The listing builds one solid part. Answer for the finished solid, in the listing's coordinates (mm). A direction names the side the tool comes from. Give positions to 0.01 mm unless a question says otherwise; leave off trailing zeros. Loops run counter-clockwise (first coordinate to the right, second up) from the corner with the lowest first, then second, coordinate; pieces in that order, holes last. Notation, with made-up numbers: M 13,61.25 L 60,61.25 A8 ccw 60,73.25 Z; hole C -0.75,-24 d1. An arc over 180 degrees is marked long. One line per item, written item: value. Start each with the question number.
Q1. Consider L1, parallel to X at y = 1.6, z = -3.75; L2, parallel to Y at x = 3, z = 7.5; L3, parallel to Y at x = -5.75, z = -0.25. Determine where each line is inside the solid, lowest interval first.
Q2. The mould has two halves that part along X. Classify faces 1 (the flat face through (8, 3, -3)), 2 (the cylindrical face through (4.579, 0.641, -5.356)), 3 (the flat face through (8.5, 2, -1)), 4 (the cylindrical face through (0, 1.8, 3.4)): +X half, -X half, draft (parallel to the pull), parting line (faces both ways), or undercut.
Q3. A cutting plane is placed at A-A, the plane y = 2.1. Determine the outline of the cut face in (x, z), and give its area (3 significant figures).
Q4. A cutting plane is placed at D-D, the plane x = -3. Determine the outline of the cut face in (y, z), and give its area (3 significant figures).
Q5. For faces 5 (the flat face through (0, 2, -8.5)), 6 (the flat face through (-8, 3, -3)), 7 (the flat face through (5, 0, -6)), 8 (the cylindrical face through (-6.421, 0.641, 6.144)), 9 (the cylindrical face through (0, 3, -8)), determine the directions among +Z, -Z, +X, -X, +Y, -Y from which every point of the face is accessible in a straight line to the end or side of a thin tool.
Q6. A cutting plane is placed at B-B, the plane x = 0. Determine the outline of the cut face in (y, z).
Q7. A cutting plane is placed at C-C, the plane z = 5.5. Determine the outline of the cut face in (x, y), and give its area (3 significant figures).
Q8. Flat-ended cylindrical pins translate along their axes: pin 1 (1 mm diameter, centred on x = -2.5, z = -6.5, fed in from -Y); pin 2 (4.5 mm diameter, centred on x = -3.5, z = 4.5, fed in from +Y); pin 3 (1.2 mm diameter, centred on x = -8, y = 3, fed in from +Z). Find the tip coordinate at first contact, or state that the pin passes through.
from build123d import *

# Parameters (mm, degrees)
SKETCH1_W           = 17
SKETCH1_H           = 17
BOSS_EXTRUDE1_DEPTH = 3.5
CUT_EXTRUDE1_DEPTH  = 4.5
CUT_EXTRUDE2_DEPTH  = 0.6
SKETCH5_W           = 17
SKETCH5_H           = 6
CUT_EXTRUDE3_DEPTH  = 0.6
SKETCH6_R           = 8
CUT_EXTRUDE4_DEPTH  = 1.2
SKETCH7_OUTSIDE_W   = 23.86
SKETCH7_OUTSIDE_H   = 23.86
SKETCH7_OUTSIDE_R   = 1.25
CUT_EXTRUDE5_DEPTH  = 1.3
CUT_EXTRUDE6_DEPTH  = 1
BOSS_EXTRUDE4_DEPTH = 1


with BuildPart() as part:
    # Sketch1 → Boss-Extrude1 (new body)
    with BuildSketch(Plane(origin=(0, 0, 0), x_dir=(1, 0, 0), z_dir=(0, 1, 0))):
        Rectangle(SKETCH1_W, SKETCH1_H)
    extrude(amount=BOSS_EXTRUDE1_DEPTH)

    # Sketch2 → Cut-Extrude1 (cut, through all)
    with BuildSketch(Plane(origin=(0, 3.5, 0), x_dir=(1, 0, 0), z_dir=(0, 1, 0))):
        Polygon((-8.5, -5.812994231), (-5.812994231, -8.5), (-8.5, -8.5), align=None)
    cut_extrude1 = extrude(amount=-CUT_EXTRUDE1_DEPTH, mode=Mode.SUBTRACT)

    # Mirror1: Cut-Extrude1 across plane
    add(cut_extrude1.mirror(Plane(origin=(0, 0, 0), x_dir=(0, 0, 1), z_dir=(1, 0, 0))), mode=Mode.SUBTRACT)

    # Sketch3 → Cut-Extrude2 (cut)
    with BuildSketch(Plane(origin=(0, 3.5, 0), x_dir=(1, 0, 0), z_dir=(0, 1, 0))):
        Polygon((-8.5, 3), (8.5, 3), (8.5, -5.812994231), (5.812994231, -8.5), (-5.812994231, -8.5), (-8.5, -5.812994231), align=None)
    extrude(amount=-CUT_EXTRUDE2_DEPTH, mode=Mode.SUBTRACT)

    # Sketch5 → Cut-Extrude3 (cut)
    with BuildSketch(Plane(origin=(0, 2.9, 0), x_dir=(1, 0, 0), z_dir=(0, 1, 0))):
        Rectangle(SKETCH5_W, SKETCH5_H)
    extrude(amount=-CUT_EXTRUDE3_DEPTH, mode=Mode.SUBTRACT)

    # Sketch6 → Cut-Extrude4 (cut)
    with BuildSketch(Plane(origin=(0, 3.5, 0), x_dir=(1, 0, 0), z_dir=(0, 1, 0))):
        Circle(SKETCH6_R)
    extrude(amount=-CUT_EXTRUDE4_DEPTH, mode=Mode.SUBTRACT)

    # Sketch7 outside → Cut-Extrude5 (cut)
    with BuildSketch(Plane.XZ):
        Rectangle(SKETCH7_OUTSIDE_W, SKETCH7_OUTSIDE_H)
        with Locations((-5.5, -6.20094747)):
            Circle(SKETCH7_OUTSIDE_R, mode=Mode.SUBTRACT)
        with Locations((-5.5, 5.29905253)):
            Circle(SKETCH7_OUTSIDE_R, mode=Mode.SUBTRACT)
        with Locations((5.5, 5.29905253)):
            Circle(SKETCH7_OUTSIDE_R, mode=Mode.SUBTRACT)
        with Locations((5.5, -6.20094747)):
            Circle(SKETCH7_OUTSIDE_R, mode=Mode.SUBTRACT)
    extrude(amount=-CUT_EXTRUDE5_DEPTH, mode=Mode.SUBTRACT)

    # Sketch8 → Cut-Extrude6 (cut)
    with BuildSketch(Plane.XZ.offset(-1.3)):
        with BuildLine():
            Line((-0.6, -8.5), (0.6, -8.5))
            Line((0.6, -8.5), (0.749551834, -4.175923885))
            ThreePointArc((0.749551834, -4.175923885), (0, -3.4), (-0.749551834, -4.175923885))
            Line((-0.749551834, -4.175923885), (-0.6, -8.5))
        make_face()
    cut_extrude6 = extrude(amount=-CUT_EXTRUDE6_DEPTH, mode=Mode.SUBTRACT)

    # Mirror2: Cut-Extrude6 across plane
    add(cut_extrude6.mirror(Plane.XY), mode=Mode.SUBTRACT)

    # Sketch11 → Boss-Extrude4 (add)
    with BuildSketch(Plane.XZ.offset(-1.3)):
        Polygon((-0.6, -8.5), (0.6, -8.5), (0.634585847, -7.5), (-0.634585847, -7.5), align=None)
    boss_extrude4 = extrude(amount=-BOSS_EXTRUDE4_DEPTH)

    # Mirror3: Boss-Extrude4 across plane
    add(boss_extrude4.mirror(Plane.XY))


solid = part.part
Answer block:
1. L1: -8.5 to -0.63, 0.63 to 8.5
1. L2: 1.3 to 2.9
1. L3: 1.3 to 2.3
2. face 1: draft
2. face 2: undercut
2. face 3: +X half
2. face 4: undercut
3. outline: M -8.5,-8.5 L 8.5,-8.5 L 8.5,5.81 L 5.81,8.5 L -5.81,8.5 L -8.5,5.81 Z; hole M -0.75,-4.18 L -0.63,-7.5 L 0.63,-7.5 L 0.75,-4.18 A0.75 ccw long Z; hole M -0.75,4.18 A0.75 ccw long 0.75,4.18 L 0.63,7.5 L -0.63,7.5 Z
3. area: 271 mm^2
4. outline: M 1.3,-8.5 L 3.5,-8.5 L 3.5,-7.42 L 2.3,-7.42 L 2.3,7.42 L 2.9,7.42 L 2.9,8.5 L 1.3,8.5 Z
4. area: 19.0 mm^2
5. face 5: -Z, +X, -X, +Y, -Y
5. face 6: +X, -X, +Y
5. face 7: +Z, -Z, +X, -X, -Y
5. face 8: -Y
5. face 9: +Y
6. outline: M 1.3,-8.5 L 3.5,-8.5 L 3.5,-8 L 2.3,-8 L 2.3,-7.5 L 1.3,-7.5 Z; M 1.3,-3.4 L 2.3,-3.4 L 2.3,3.4 L 1.3,3.4 Z; M 1.3,7.5 L 2.3,7.5 L 2.3,8 L 2.9,8 L 2.9,8.5 L 1.3,8.5 Z
7. outline: M -8.5,1.3 L -6.73,1.3 L -6.73,0 L -4.27,0 L -4.27,1.3 L -0.7,1.3 L -0.7,2.3 L -5.81,2.3 L -5.81,2.9 L -8.5,2.9 Z; M 0.7,1.3 L 4.27,1.3 L 4.27,0 L 6.73,0 L 6.73,1.3 L 8.5,1.3 L 8.5,2.9 L 5.81,2.9 L 5.81,2.3 L 0.7,2.3 Z
7. area: 25.2 mm^2
8. pin 1: y = 1.3
8. pin 2: y = 2.3
8. pin 3: z = 6.9
